Design review of the part built by this model. Coordinates are the model's own, in mm. Coordinates: 2 decimals unless noted, no trailing zeros. Write each loop counter-clockwise with the first axis right and the second up, starting at its lowest first coordinate (ties: lowest second). Pieces come first, ordered by that corner, then holes. Notation, with made-up numbers: (69.25, 72.5) -> (92.25, 72.5) arc R16 ccw to (92.25, 95.5) -> close; hole circle Ø10 at (18, 36). An arc over 180 degrees is marked (long way). Answer in a Markdown table with one row per item. Add a question column.
Item 1: Clearance check with flat-ended pins moving along their axes: P1, Ø3, axis at x = 46.5, z = 1.5, coming from the -Y side; P2, Ø3, axis at y = 86.5, z = 1.5, coming from the +X side; P3, Ø2, axis at x = -20.5, y = -17, coming from the -Z side; P4, Ø2, axis at x = 50.5, z = 2, coming from the -Y side. State where each tip first meets the part, or that it passes through.
Item 2: Take a section at A-A, the plane z = 3.35. Write out the cut boundary in (x, y), and give its area (3 significant figures).
Item 3: Take a section at C-C, the plane x = 28.5. Write out the cut boundary in (y, z), and give its area (3 significant figures).
Item 4: Take a section at D-D, the plane y = 37. Write out the cut boundary in (x, z).
Item 5: To check wall thickness, follow line 1 (Y direction, x = 28.5, z = 2.75); line 2 (X direction, y = 40, z = 2.25); line 3 (X direction, y = -8, z = 1.2). State the ranges of each line that lie inside material, in increasing order.
Item 6: Take a section at B-B, the plane y = -15. Write out the cut boundary in (x, z).
Autodesk Fusion 360 part; units mm, degrees
sketch "スケッチ1" plane through (0, 0, 0) normal (0, 0, 1) x (1, 0, 0)
  line L0 (-21.5, 91) -> (-68.5, 91)
  line L1 (-68.5, 91) -> (-68.5, -91)
  line L2 (-68.5, -91) -> (-21.5, -91)
  line L3 (68.5, -75) -> (68.5, 80)
  line L4 (60.2198, 80) -> (-68.5, -91) construction
  line L5 (-68.5, 91) -> (57.8776, -76.8884) construction
  line L6 (-21.5, 91) -> (-21.5, 80)
  line L7 (-21.5, 80) -> (68.5, 80)
  line L8 (-68.5, -91) -> (-21.5, -91) construction
  line L9 (-21.5, -91) -> (68.5, -75)
  dimension "d2" = 182
  dimension "d5" = 47
extrude "押し出し1" add sketch "スケッチ1" along normal blind 6
chamfer "面取り1" distance 15 angle 45 2 edges at (-68.5, -91, 3) (-68.5, 91, 3)
sketch "スケッチ2" plane through (0, 0, 6) normal (0, 0, 1) x (-1, 0, 0)
  line L0 (53.5, -91) -> (68.5, -76)
  line L1 (68.5, -76) -> (68.5, 76)
  line L2 (68.5, 76) -> (53.5, 91)
  line L3 (53.5, 91) -> (21.5, 91)
  line L4 (21.5, 91) -> (-68.5, 75)
  line L5 (-68.5, 75) -> (-68.5, -80)
  line L6 (-68.5, -80) -> (21.5, -80)
  line L7 (21.5, -80) -> (21.5, -91)
  line L8 (21.5, -91) -> (53.5, -91)
  line L9 (-68.5, -80) -> (-28.5, -80) construction
  line L10 (-28.5, -80) -> (-28.5, -40) construction
  line L11 (-28.5, -40) -> (-68.5, -40) construction
  line L12 (-68.5, -40) -> (-68.5, -80) construction
  line L13 (-68.5, -40) -> (-28.5, -40) construction
  line L14 (-28.5, -40) -> (-28.5, 15) construction
  line L15 (-28.5, 15) -> (-68.5, 15) construction
  line L16 (-68.5, 15) -> (-68.5, -40) construction
  point P0 (-28.5, -40)
  point P1 (-28.5, 15)
  dimension "d10" = 40
  dimension "d11" = 40
  dimension "d12" = 40
  dimension "d13" = 55
hole "穴1" at (28.5, 40, 6) at (28.5, -15, 6) direction (0, 0, -1) diameter 18 end through all
equation "d5 = 15 mm + 32 mm"
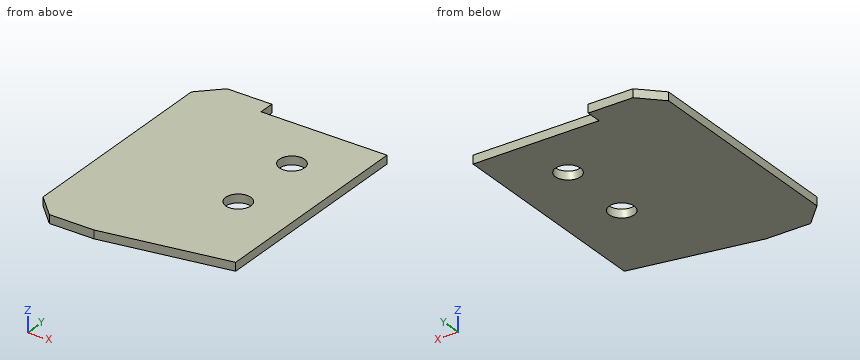
Answers:
| question | item | result |
|---|---|---|
| 1 | P1 | stops at y = -79.18 |
| 1 | P2 | stops at x = -21.5 |
| 1 | P3 | stops at z = 0 |
| 1 | P4 | stops at y = -78.38 |
| 2 | outline | (-68.5, -76) -> (-53.5, -91) -> (-21.5, -91) -> (68.5, -75) -> (68.5, 80) -> (-21.5, 80) -> (-21.5, 91) -> (-53.5, 91) -> (-68.5, 76) -> close; hole circle Ø18 at (28.5, -15); hole circle Ø18 at (28.5, 40) |
| 2 | area | 22,500 mm^2 |
| 3 | outline | (-82.11, 0) -> (-24, 0) -> (-24, 6) -> (-82.11, 6) -> close; (-6, 0) -> (31, 0) -> (31, 6) -> (-6, 6) -> close; (49, 0) -> (80, 0) -> (80, 6) -> (49, 6) -> close |
| 3 | area | 757 mm^2 |
| 4 | outline | (-68.5, 0) -> (20.01, 0) -> (20.01, 6) -> (-68.5, 6) -> close; (36.99, 0) -> (68.5, 0) -> (68.5, 6) -> (36.99, 6) -> close |
| 5 | line 1 | y = -82.11 to -24, -6 to 31, 49 to 80 |
| 5 | line 2 | x = -68.5 to 19.5, 37.5 to 68.5 |
| 5 | line 3 | x = -68.5 to 22.84, 34.16 to 68.5 |
| 6 | outline | (-68.5, 0) -> (19.5, 0) -> (19.5, 6) -> (-68.5, 6) -> close; (37.5, 0) -> (68.5, 0) -> (68.5, 6) -> (37.5, 6) -> close |
